Geometry: final body of the model. Coordinates: model frame, mm. A direction names the side the tool comes from. Round coordinates to 2 decimals unless told otherwise and drop trailing zeros. Loops run counter-clockwise (first coordinate to the right, second up) from the corner with the lowest first, then second, coordinate; pieces in that order, holes last. Notation, with made-up numbers: M 78,12.25 L 129,12.25 A15 cw 129,39.25 Z; hole C -30,8.25 d9. An arc over 180 degrees is marked long. Return JSON: item names as keys, results as strings.
from build123d import *

# Parameters (mm, degrees)
F0_W      = 457.2
F0_H      = 63.5
F1_DEPTH  = 31.75
F2_W      = 31.75
F2_H      = 63.5
F3_DEPTH  = 177.8
F4_W      = 31.75
F4_H      = 63.5
F4_W_2    = 425.45
F5_DEPTH  = 31.75
F7_DEPTH  = 254
F9_DEPTH  = 508
F10_W     = 76.2
F10_H     = 12.7
F11_DEPTH = 346.71


with BuildPart() as f1:
    # F0 (on Front) → F1 (new body)
    with BuildSketch(Plane.XZ):
        with Locations((228.6, 31.75)):
            Rectangle(F0_W, F0_H)
    extrude(amount=F1_DEPTH)

    # F2 (on face) → F3 (join)
    with BuildSketch(Plane.XZ.offset(31.75)):
        with Locations((441.325, 31.75)):
            Rectangle(F2_W, F2_H)
    extrude(amount=F3_DEPTH)

    # F4 (on face) → F5 (join)
    with BuildSketch(Plane.XZ.offset(209.55)):
        with Locations((441.325, 31.75)):
            Rectangle(F4_W, F4_H)
        with Locations((212.725, 31.75)):
            Rectangle(F4_W_2, F4_H)
    extrude(amount=F5_DEPTH)

    # F6 (on face) → F7 (cut)
    with BuildSketch(Plane.XZ.offset(241.3)):
        Polygon((180.975, 41.275), (314.325, 41.275), (314.325, 53.975), (247.65, 53.975), (180.975, 53.975), align=None)
    extrude(amount=-F7_DEPTH, mode=Mode.SUBTRACT)

    # F8 (on face) → F9 (cut)
    with BuildSketch(Plane.XZ.offset(241.3)):
        with BuildLine():
            ThreePointArc((41.269663, 47.625), (44.444663, 44.45), (47.619663, 47.625))
            ThreePointArc((47.619663, 47.625), (44.444663, 50.8), (41.269663, 47.625))
        make_face()
    extrude(amount=-F9_DEPTH, mode=Mode.SUBTRACT)

    # F10 (on face) → F11 (cut)
    with BuildSketch(Plane.XZ.offset(241.3)):
        with Locations((142.875, 47.625)):
            Rectangle(F10_W, F10_H)
    extrude(amount=-F11_DEPTH, mode=Mode.SUBTRACT)


solid = f1.part
Q1. Section query B-B (x = 63.5). Output: boundary loops of the cut face in (y, z).
Determined:
{"outline": "M -241.3,0 L -209.55,0 L -209.55,63.5 L -241.3,63.5 Z; M -31.75,0 L 0,0 L 0,63.5 L -31.75,63.5 Z"}
Q2. Section query C-C (z = 8). Output: boundary loops of the cut face in (x, y), plus the area to 3 significant figures.
Determined:
{"outline": "M 0,-241.3 L 457.2,-241.3 L 457.2,0 L 0,0 L 0,-31.75 L 425.45,-31.75 L 425.45,-209.55 L 0,-209.55 Z", "area": "34,700 mm^2"}
Q3. Pin query (flat end, axial travel): pin 1 (19 mm diameter, centred on y = -123, z = 25, fed in from -X); pin 2 (4 mm diameter, centred on x = 44.44, z = 47.62, fed in from +Y). Return the tip coordinate at first contact, or that it passes through.
Determined:
{"pin 1": "stops at x = 425.45", "pin 2": "passes through"}
Q4. Section query A-A (x = 189.5). Output: boundary loops of the cut face in (y, z) (3 decimals).
Determined:
{"outline": "M -241.3,0 L -209.55,0 L -209.55,41.275 L -241.3,41.275 Z; M -241.3,53.975 L -209.55,53.975 L -209.55,63.5 L -241.3,63.5 Z; M -31.75,0 L 0,0 L 0,41.275 L -31.75,41.275 Z; M -31.75,53.975 L 0,53.975 L 0,63.5 L -31.75,63.5 Z"}
Q5. Material intervals for L1, parallel to Y at x = 20, z = 14.5; L2, parallel to X at y = -207, z = 27; L3, parallel to Z at x = 189.5, y = -17 (3 decimals), sorted ascending.
Determined:
{"L1": "y = -241.3 to -209.55, -31.75 to 0", "L2": "x = 425.45 to 457.2", "L3": "z = 0 to 41.275, 53.975 to 63.5"}
Q6. Pull-direction query (Z, two-part tool) for faces 1 (the flat face through (208, -16, 41.275)), 2 (the flat face through (210, -31.75, 32)), 3 (the flat face through (264, -31, 63.5)); classes: pulls with the +Z half, pulls with the -Z half, needs draft (parallel to the pull), parting line crosses it, or undercut.
Determined:
{"face 1": "undercut", "face 2": "needs draft", "face 3": "pulls with the +Z half"}
Q7. Reachability of faces 4 (the flat face through (208, -226, 41.275)), 5 (the flat face through (0, -225, 31)), 6 (the flat face through (210, -209.55, 32)) from +Z, -Z, +X, -X, +Y, -Y: full face, straight path, thin tool, end or side. Return the list, or none.
Determined:
{"face 4": "+Y, -Y", "face 5": "+Z, -Z, -X, +Y, -Y", "face 6": "+Z, -Z, -X"}
Q8. Section query D-D (y = -49.5). Output: boundary loops of the cut face in (x, z).
Determined:
{"outline": "M 425.45,0 L 457.2,0 L 457.2,63.5 L 425.45,63.5 Z"}
